For this review, use the dimensioned drawing (mm, ordinates from the lowest corner) and the shaded views. Coordinates: 2 decimals unless noted, no trailing zeros. Write each loop counter-clockwise with the first axis right and the second up, starting at its lowest first coordinate (ties: lowest second). Pieces come first, ordered by that corner, then holes. Notation, with made-up numbers: (-3, 18) -> (26, 18) arc R15 cw to (26, 22) -> close; hole circle Ø3 at (-21.75, 70). An arc over 180 degrees is marked (long way). Put each result on its own line as item: value. Start each with the question number.
Item 1: Insertion check: P1, Ø4, axis at x = 8, y = 86, coming from the -Z side; P2, Ø2, axis at x = 8, y = 46, coming from the +Z side. Each pin has a flat end and moves straight along its axis. Give the tip position at first contact, or say it passes through.
Item 2: Consider section A-A on y = 106. Give the boundary of the cut face in (x, z).
Item 3: To check wall thickness, follow L1, parallel to Y at x = 48, z = 1.65; L2, parallel to X at y = 96, z = 2; L3, parallel to X at y = 126.5, z = 0.2. State the ranges of each line that lie inside material, in increasing order.
Item 4: Consider section C-C on z = 0.45. Give the number of separate pieces and of enclosed holes in the cut face, and give its area (3 significant figures).
Item 5: Consider section B-B on x = 38. Give the boundary of the cut face in (y, z), and give its area (3 significant figures).
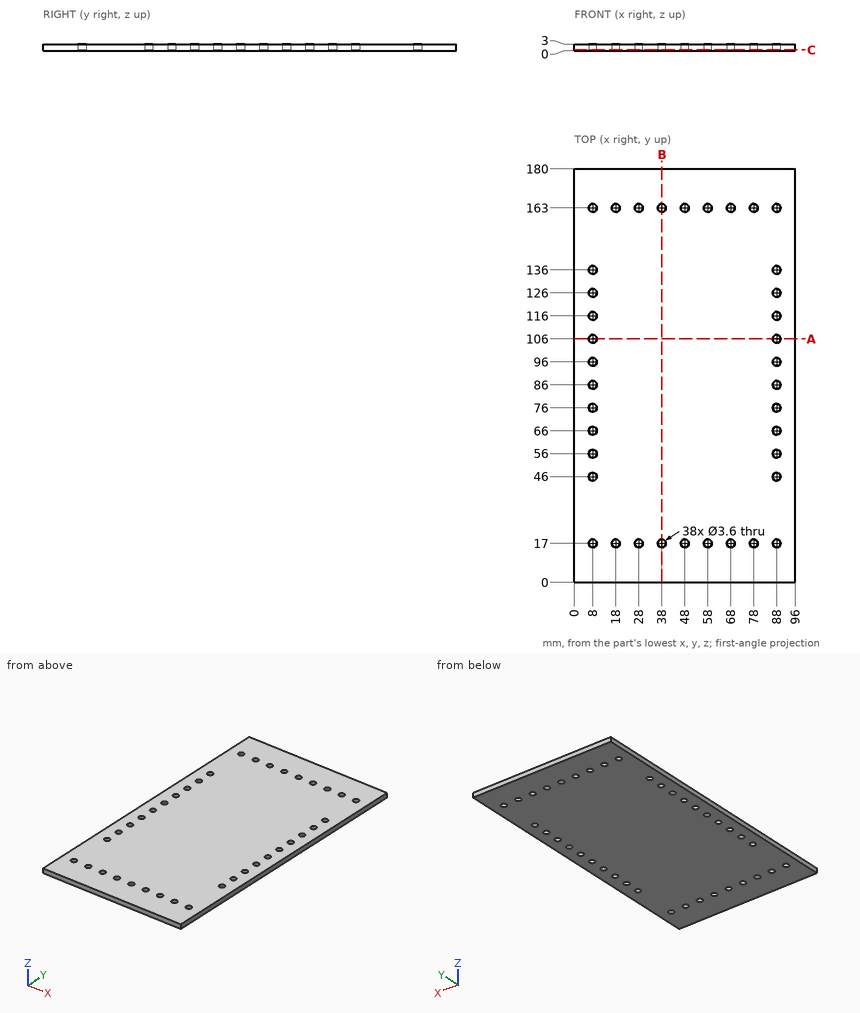
Return value:
1. P1: z = 0
1. P2: through
2. outline: (0, 0) -> (6.2, 0) -> (6.2, 3) -> (0, 3) -> close; (9.8, 0) -> (86.2, 0) -> (86.2, 3) -> (9.8, 3) -> close; (89.8, 0) -> (96, 0) -> (96, 3) -> (89.8, 3) -> close
3. L1: 0 to 15.2, 18.8 to 161.2, 164.8 to 180
3. L2: 0 to 6.2, 9.8 to 86.2, 89.8 to 96
3. L3: 0 to 6.27, 9.73 to 86.27, 89.73 to 96
4. separate pieces: 1
4. enclosed holes: 38
4. area: 16,900 mm^2
5. outline: (0, 0) -> (15.2, 0) -> (15.2, 3) -> (0, 3) -> close; (18.8, 0) -> (161.2, 0) -> (161.2, 3) -> (18.8, 3) -> close; (164.8, 0) -> (180, 0) -> (180, 3) -> (164.8, 3) -> close
5. area: 518 mm^2
